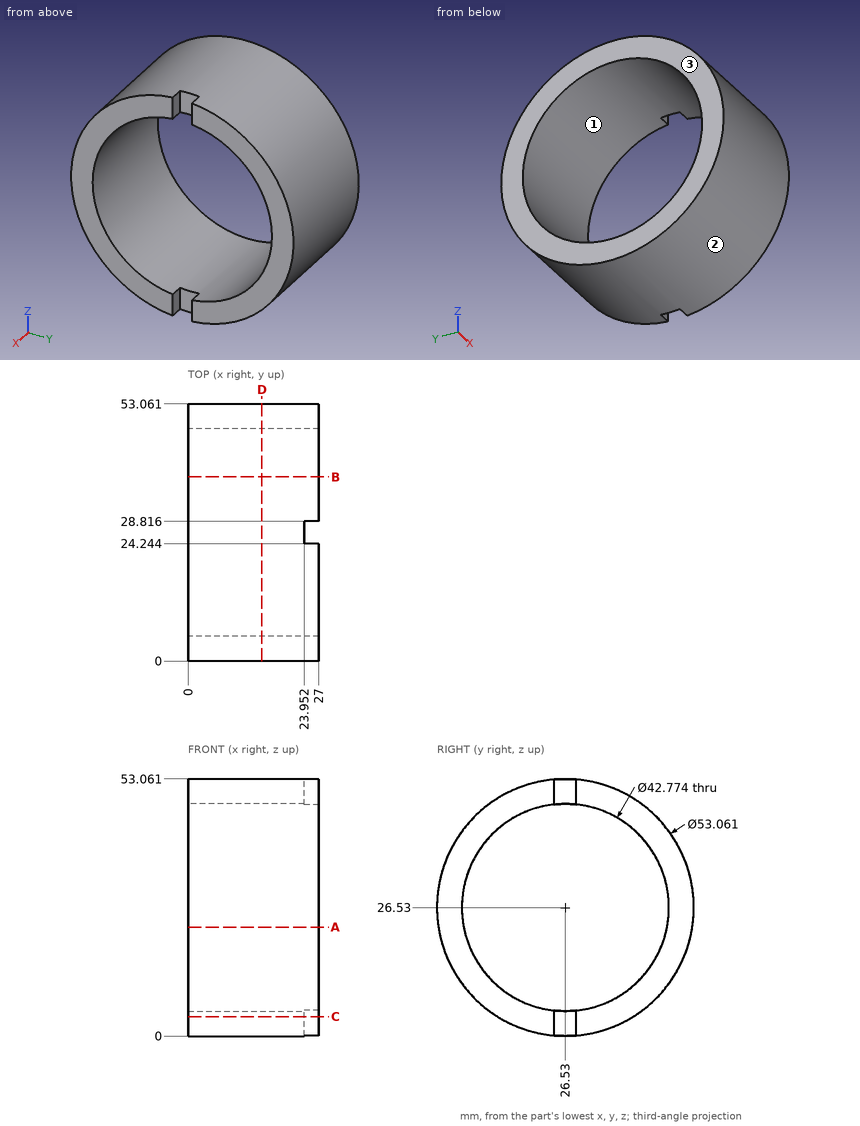
The drawing under review shows one solid part. Ordinate dimensions are in mm from its lowest x, y, z. Round coordinates to 2 decimals unless told otherwise and drop trailing zeros. Order: outer loops, then holes, each group sorted by start corner. A loop starts at its lowest first (then second) coordinate and runs counter-clockwise, first axis right, second up. Notation, with made-up numbers: (39, 84.25) - (88, 84.25) arc R20 ccw to (88, 122.25) - close; hole circle Ø3 at (46, 3). An arc over 180 degrees is marked (long way). Return JSON: item names as keys, results as strings.
Q1. For pin 1 Ø1 at (x, y) = (16, 34.5) entering from -Z; pin 2 Ø6 at (x, y) = (15, 42.5) entering from +Z (1 decimal); pin 3 Ø1.5 at (x, z) = (26, 50) entering from -Y; pin 4 Ø1 at (y, z) = (7, 24.5) entering from +X, all flat-tipped, find the tip position at first contact; note any pin that passes through.
Computed values:
{"pin 1": "stops at z = 1.07", "pin 2": "stops at z = 49.7", "pin 3": "stops at y = 12.83", "pin 4": "passes through"}
Q2. Consider section D-D on x = 15.25. Write out the cut boundary in (y, z).
Computed values:
{"outline": "circle Ø53.06 at (26.53, 26.53); hole circle Ø42.77 at (26.53, 26.53)"}
Q3. Consider section A-A on z = 22.5. Write out the cut boundary in (x, y), plus the area to 3 significant figures.
Computed values:
{"outline": "(0, 0.31) - (27, 0.31) - (27, 5.53) - (0, 5.53) - close; (0, 47.53) - (27, 47.53) - (27, 52.75) - (0, 52.75) - close", "area": "282 mm2"}
Q4. Wall thickness on L1, parallel to Z at x = 18, y = 27; L2, parallel to Z at x = 8.5, y = 32 (1 decimal); L3, parallel to Y at x = 2.5, z = 17 (1 decimal): over which ranges is each line inside the solid? List them lowest first. Write a range as [from, to].
Computed values:
{"L1": "z = [0, 5.15], [47.91, 53.06]", "L2": "z = [0.6, 5.9], [47.2, 52.5]", "L3": "y = [1.8, 7.4], [45.7, 51.3]"}
Q5. Consider section C-C on z = 4. Write out the cut boundary in (x, y) (1 decimal).
Computed values:
{"outline": "(0, 12.5) - (27, 12.5) - (27, 24.2) - (24, 24.2) - (24, 28.8) - (27, 28.8) - (27, 40.5) - (0, 40.5) - close"}
Q6. Consider section B-B on y = 38. Write out the cut boundary in (x, z), plus the area to 3 significant figures.
Computed values:
{"outline": "(0, 2.61) - (27, 2.61) - (27, 8.48) - (0, 8.48) - close; (0, 44.58) - (27, 44.58) - (27, 50.45) - (0, 50.45) - close", "area": "317 mm2"}
Q7. The part is to be moulded in two halves that separate along Z. For the marked faces 1, 2 and 3, say which applies: pulls with the +Z half, pulls with the -Z half, needs draft (parallel to the pull), parting line crosses it, or undercut.
Computed values:
{"face 1": "undercut", "face 2": "parting line crosses it", "face 3": "needs draft"}
